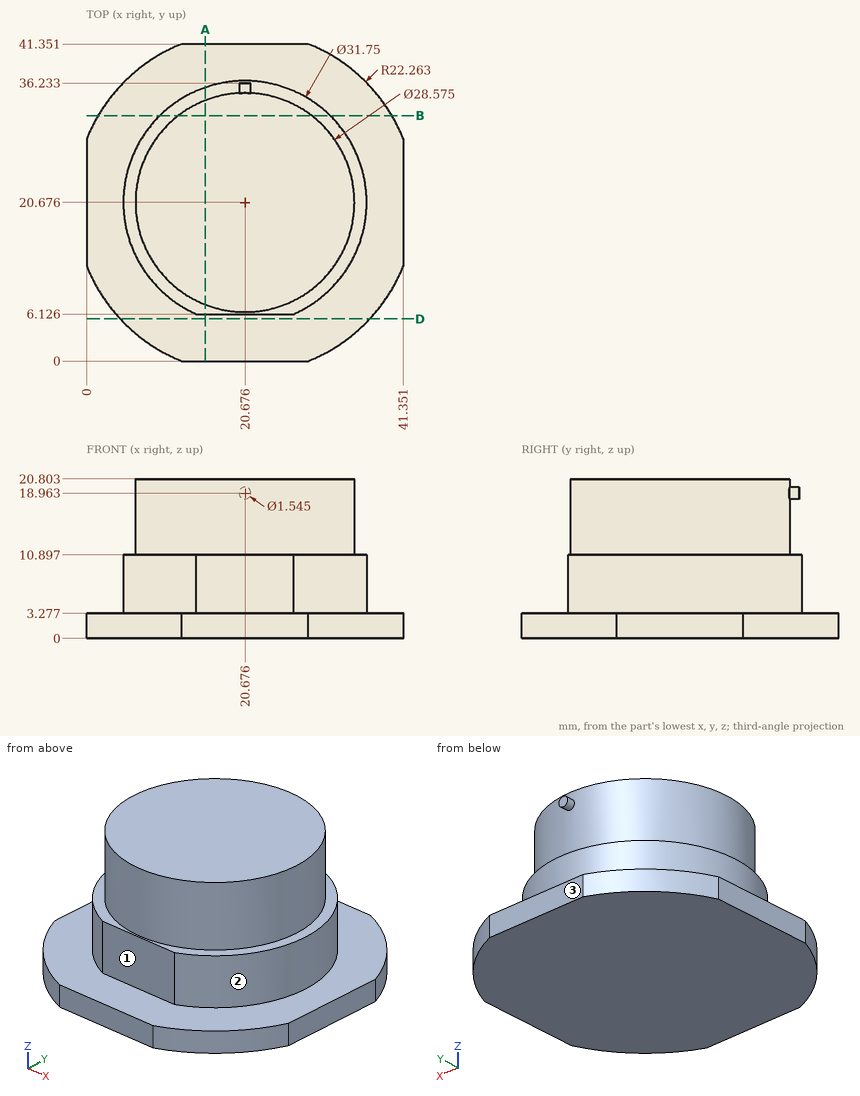
Can you work these out from the drawing? Everything is in mm from the part's minimum corner. A direction names the side the tool comes from. Coordinates: 2 decimals unless noted, no trailing zeros. Loops run counter-clockwise (first coordinate to the right, second up) from the corner with the lowest first, then second, coordinate; pieces in that order, holes last.
1. For the marked faces 1, 2 and 3, which set-ups out of +Z, -Z, +X, -X, +Y, -Y let a thin tool reach every point of the face, with its end or its side?
2. I need wall thicknesses on L1, parallel to Z at x = 31, y = 6; L2, parallel to Y at x = 21, z = 10; L3, parallel to Y at x = 21, z = 20. Which ranges of each line are inside material? Lowest first, please.
3. Imagine slicing it at D-D, the plane y = 5.5. Please give me the cut outline in (x, z) (1 decimal), and give its area (3 significant figures).
4. Imagine slicing it at A-A, the plane x = 15.5. Please give me the cut outline in (y, z).
5. For P1, Ø2, axis at x = 11, z = 2.5, coming from the +Y side; P2, Ø10, axis at x = 6, z = 17, coming from the +Y side; P3, Ø0.5, axis at x = 20.5, z = 19, coming from the +Y side, each with a flat end and sliding along its axis, tell me the tip position at first contact or that it passes through.
6. Imagine slicing it at B-B, the plane y = 32. Please give me the cut outline in (x, z).
Taken from the geometry:
1. face 1: +Z, +X, -X, -Y
1. face 2: +Z
1. face 3: +Z, -Z, +X, -X, +Y
2. L1: z = 0 to 3.28
2. L2: y = 6.13 to 36.55
2. L3: y = 6.39 to 34.96
3. outline: (4.4, 0) - (37, 0) - (37, 3.3) - (4.4, 3.3) - close
3. area: 107 mm2
4. outline: (0, 0) - (41.35, 0) - (41.35, 3.28) - (35.68, 3.28) - (35.68, 10.9) - (33.99, 10.9) - (33.99, 20.8) - (7.36, 20.8) - (7.36, 10.9) - (6.13, 10.9) - (6.13, 3.28) - (0, 3.28) - close
5. P1: stops at y = 41.18
5. P2: stops at y = 31.19
5. P3: stops at y = 36.23
6. outline: (1.51, 0) - (39.84, 0) - (39.84, 3.28) - (31.8, 3.28) - (31.8, 10.9) - (29.39, 10.9) - (29.39, 20.8) - (11.96, 20.8) - (11.96, 10.9) - (9.55, 10.9) - (9.55, 3.28) - (1.51, 3.28) - close
